Print and shaded views of the part. All mm, measured from the part's lowest x, y and z. A direction names the side the tool comes from. Round coordinates to 2 decimals unless told otherwise and drop trailing zeros. Loops run counter-clockwise (first coordinate to the right, second up) from the corner with the lowest first, then second, coordinate; pieces in that order, holes last. Notation, with made-up numbers: (-29.5, 55.25) - (-7.5, 55.25) arc R21 cw to (-7.5, 91.25) - close; hole circle Ø10 at (0, 86.5). An arc over 180 degrees is marked (long way). Use one line per item in the form item = value. Start each with the question number.
Q1. Saw through at B-B (y = 30). Give the cut face in (x, z), then the cut area to 3 significant figures.
Q2. Saw through at C-C (x = 25.5). Give the cut face in (y, z).
Q3. Pin check, flat tips, straight feed: pin 1 (1.5 mm diameter, centred on x = 44, z = 7.5, fed in from +Y); pin 2 (10 mm diameter, centred on x = 22, z = 13, fed in from +Y); pin 3 (8 mm diameter, centred on x = 28, z = 6, fed in from +Y). Stop position of each tip, or through.
Q4. Saw through at A-A (z = 1.75). Give the cut face in (x, y), then the cut area to 3 significant figures.
Q5. Saw through at D-D (z = 12.5). Give the cut face in (x, y).
Q6. Drill centre lines: line 1 (Y direction, x = 30, z = 4.25); line 2 (Y direction, x = 51, z = 4.5) (1 decimal); line 3 (X direction, y = 29.5, z = 6). Where is each one in solid material? Low to high.
Q7. Mould opens along Y. For the marked faces 3, 4 and 5 say: released by +Y, released by -Y, zero draft, split by the parting line, or undercut.
Q8. 3-axis set-ups, long thin cutter, end or side, ignore diameter. For the marked faces 1 and 2: which of +Z, -Z, +X, -X, +Y, -Y reach the whole face in a straight line?
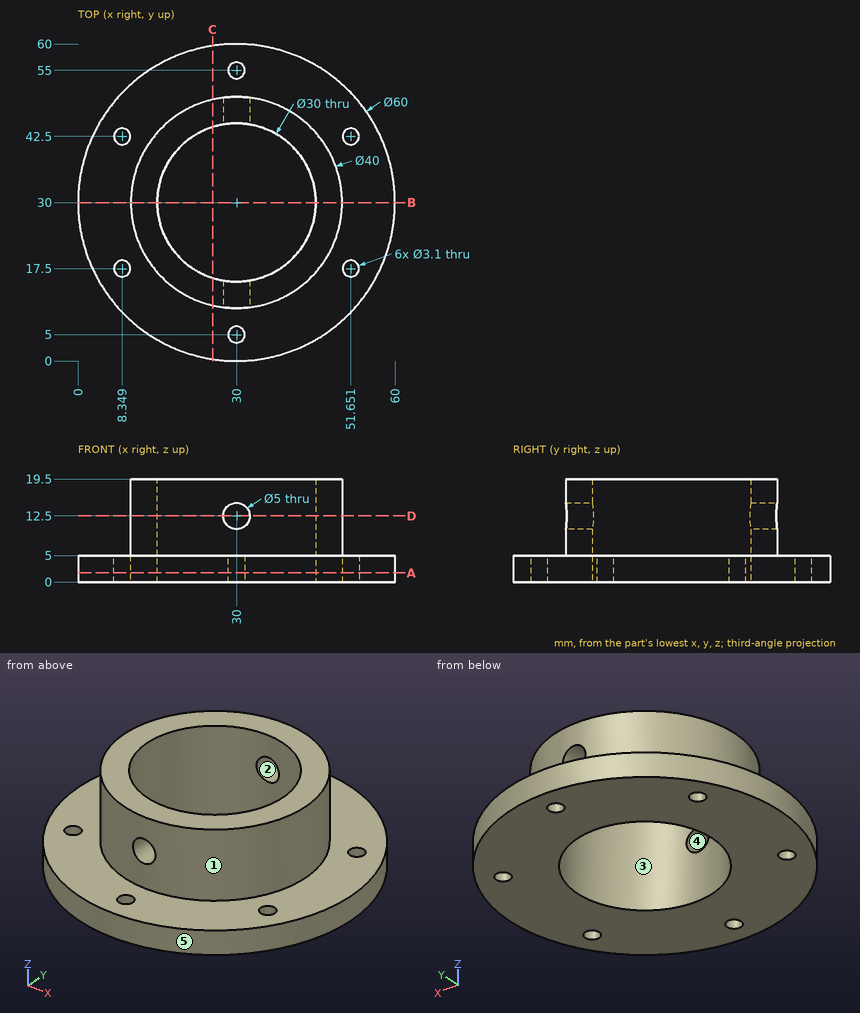
Report:
q1.outline = (0, 0) - (15, 0) - (15, 19.5) - (10, 19.5) - (10, 5) - (0, 5) - close; (45, 0) - (60, 0) - (60, 5) - (50, 5) - (50, 19.5) - (45, 19.5) - close
q1.area = 295 mm²
q2.outline = (0.34, 0) - (15.69, 0) - (15.69, 19.5) - (10.51, 19.5) - (10.51, 5) - (0.34, 5) - close; (44.31, 0) - (59.66, 0) - (59.66, 5) - (49.49, 5) - (49.49, 19.5) - (44.31, 19.5) - close
q3.pin_1 = 44.98
q3.pin_2 = 49.77
q3.pin_3 = 60
q4.outline = circle Ø60 at (30, 30); hole circle Ø3.1 at (8.35, 17.5); hole circle Ø3.1 at (8.35, 42.5); hole circle Ø30 at (30, 30); hole circle Ø3.1 at (30, 5); hole circle Ø3.1 at (30, 55); hole circle Ø3.1 at (51.65, 17.5); hole circle Ø3.1 at (51.65, 42.5)
q4.area = 2,080 mm²
q5.outline = (27.5, 10.16) - (27.5, 15.21) arc R15 cw to (27.5, 44.79) - (27.5, 49.84) arc R20 ccw to start; (32.5, 10.16) arc R20 ccw to (32.5, 49.84) - (32.5, 44.79) arc R15 cw to (32.5, 15.21) - close
q6.line_1 = 0 to 3.45, 6.55 to 15, 45 to 53.45, 56.55 to 60
q6.line_2 = 8.6 to 16.1, 18.9 to 41.1, 43.9 to 51.4
q6.line_3 = 10.01 to 15.01, 44.99 to 49.99
q7.face_3 = undercut
q7.face_4 = zero draft
q7.face_5 = split by the parting line
q8.face_1 = +Z
q8.face_2 = +Y, -Y
